Can you work these out from the model? Positions are in its coordinate system, mm. A direction names the side the tool comes from. Coordinates: 2 decimals unless noted, no trailing zeros. Order: outer loops, then holes, each group sorted by start corner. A loop starts at its lowest first (then second) coordinate and runs counter-clockwise, first axis right, second up. Notation, with made-up numbers: (58, 69) - (84, 69) arc R19 ccw to (84, 104) - close; hole circle Ø8 at (23.5, 15.5). An arc over 180 degrees is marked (long way). Return JSON: item names as keys, results as strings. Group by question number.
1) For pin 1 Ø2 at (y, z) = (3, -22) entering from +X; pin 2 Ø3.5 at (x, y) = (13.5, 3) entering from -Z; pin 3 Ø3 at (y, z) = (3.5, -11) entering from +X, each with a flat end and sliding along its axis, tell me the tip position at first contact or that it passes through.
2) Imagine slicing it at D-D (x = 37). Write out the boundary of the cut face in (y, z), and give its area (3 significant figures).
3) Imagine slicing it at C-C (x = 16). Write out the boundary of the cut face in (y, z), and give its area (3 significant figures).
4) Which directions (+Z, -Z, +X, -X, +Y, -Y) give clear straight access to the entire face, cutting with the end or side of a thin tool? Please do faces 4 (the face through (6.204, 3.451, -29.935)), 5 (the face through (21, 7, -19)).
5) If I drill on line 1 along Z through (x, y) = (19, 5); line 2 along Z through (x, y) = (28, 2); line 3 along X through (y, z) = (0.5, -12), over which ranges is the centre line in solid material (lowest first)?
6) Imagine slicing it at B-B (z = -17.5). Write out the boundary of the cut face in (x, y).
7) If we mould it in two halves opening along X, with no side actions, what happens to faces 1 (the face through (22, 3, -23)), 2 (the face through (18.82, 3.45, -19.11)), 3 (the face through (23, 3, 0))? For each: pulls with the +X half, pulls with the -X half, needs draft (parallel to the pull), parting line crosses it, or undercut.
8) Imagine slicing it at A-A (y = 3.5). Write out the boundary of the cut face in (x, z), and give its area (3 significant figures).
```python
from build123d import *

# Parameters (mm, degrees)
BOSS_EXTRUDE1_DEPTH = 7


with BuildPart() as part:
    # Sketch1 → Boss-Extrude1 (new body)
    with BuildSketch(Plane(origin=(0, 0, 0), x_dir=(1, 0, 0), z_dir=(0, 1, 0))):
        Polygon((0, 0), (0, 45), (45, 0), align=None)
        with BuildLine():
            Line((5, 7), (5, 28.100505063))
            ThreePointArc((5, 28.100505063), (6.234633135, 29.948264128), (8.414213562, 29.514718626))
            Line((8.414213562, 29.514718626), (29.514718626, 8.414213562))
            ThreePointArc((29.514718626, 8.414213562), (29.948264128, 6.234633135), (28.100505063, 5))
            Line((28.100505063, 5), (7, 5))
            ThreePointArc((7, 5), (5.585786438, 5.585786438), (5, 7))
        make_face(mode=Mode.SUBTRACT)
    extrude(amount=BOSS_EXTRUDE1_DEPTH)


solid = part.part
```
Calculated:
{
 "1": {"pin 1": "x = 24", "pin 2": "z = -33.25", "pin 3": "x = 35.5"},
 "2": {"outline": "(0, -8) - (7, -8) - (7, 0) - (0, 0) - close", "area": "56.0 mm2"},
 "3": {"outline": "(0, -29) - (7, -29) - (7, -21.93) - (0, -21.93) - close; (0, -5) - (7, -5) - (7, 0) - (0, 0) - close", "area": "84.5 mm2"},
 "4": {"face 4": "+Y, -Y", "face 5": "+Z, -Z, +X, -X, +Y"},
 "5": {"line 1": "-26 to -18.93, -5 to 0", "line 2": "-17 to -9.93, -5 to 0", "line 3": "0 to 5, 25.93 to 33"},
 "6": {"outline": "(0, 0) - (5, 0) - (5, 7) - (0, 7) - close; (20.43, 0) - (27.5, 0) - (27.5, 7) - (20.43, 7) - close"},
 "7": {"face 1": "pulls with the +X half", "face 2": "undercut", "face 3": "needs draft"},
 "8": {"outline": "(0, -45) - (45, 0) - (0, 0) - close; hole (5, -28.1) arc R2 ccw to (8.41, -29.51) - (29.51, -8.41) arc R2 ccw to (28.1, -5) - (7, -5) arc R2 ccw to (5, -7) - close", "area": "633 mm2"}
}
